Work out the finished part from the listing and answer in its coordinate system (mm). A direction names the side the tool comes from. Coordinates: 2 decimals unless noted, no trailing zeros. Loops run counter-clockwise (first coordinate to the right, second up) from the corner with the lowest first, then second, coordinate; pieces in that order, holes last. Notation, with made-up numbers: (68.5, 87) - (121.5, 87) arc R25 cw to (121.5, 110) - close; hole circle Ø11 at (6, 18.5). An arc over 180 degrees is marked (long way). Write each question's results on one line, items separated by ' | '. Start each with the question number.
Item 1: Section A-A, the plane y = 44 is taken. Write down the section's boundary in (x, z).
Item 2: Consider probe 1 along X at (y, z) = (36, 2.5); probe 2 along Z at (x, y) = (34.5, 22); probe 3 along Y at (x, z) = (28.5, 3.75). Determine where each line is inside the solid, lowest interval first. Write a range as [from, to].
Item 3: Each of these flat-tipped pins is pushed along its axis until it touches: pin 1 Ø6 at (x, y) = (-7, 9) entering from +Z; pin 2 Ø0.9 at (y, z) = (1.5, 3.5) entering from +X; pin 3 Ø0.9 at (y, z) = (1.5, 3.5) entering from -X. Where does it stop, or does it pass through?
Item 4: Section B-B, the plane z = 6 is taken. Write down the section's boundary in (x, y).
Item 5: For a pull along Z with two mould halves and no side action, classify faces 5 (the face through (17, 29, 2)), 6 (the face through (17, 30, 0)), 7 (the face through (17, 58, 3)), 8 (the face through (46, 24, 6)) as +Z half, -Z half, draft (parallel to the pull), parting line (faces both ways), or undercut.
Item 6: Section D-D, the plane z = 1.25 is taken. Write down the section's boundary in (x, y).
Item 7: Section C-C, the plane x = 27 is taken. Write down the section's boundary in (y, z).
Item 8: A tool of negligible diameter and unlimited length cuts with its end or side. For faces 1 (the face through (45, 39, 4.7)), 2 (the face through (0, 2, 3)), 3 (the face through (17, 60, 2)), 4 (the face through (46, 55, 6)), from which of +Z, -Z, +X, -X, +Y, -Y can it reach the whole face along a straight path? Write none if from no direction.
from build123d import *

# Parameters (mm, degrees)
P_IDAT_VYSUNUT_M1_DEPTH = 2
P_IDAT_VYSUNUT_M2_DEPTH = 3
P_IDAT_VYSUNUT_M3_DEPTH = 2


with BuildPart() as part:
    # Skica1 → Přidat vysunutím1 (new body)
    with BuildSketch(Plane.XY):
        Polygon((0, 0), (34, 0), (47, 20), (47, 60), (-13, 60), (-13, 20), align=None)
    extrude(amount=P_IDAT_VYSUNUT_M1_DEPTH)

    # Skica2 → Přidat vysunutím2 (add)
    with BuildSketch(Plane.XY.offset(2)):
        Polygon((-11, 20.592880136), (0, 3.669803213), (0, 0), (-13, 20), (-13, 60), (47, 60), (47, 20), (34, 0), (34, 3.669803213), (45, 20.592880136), (45, 58), (-11, 58), align=None)
    extrude(amount=P_IDAT_VYSUNUT_M2_DEPTH)

    # Skica3 → Přidat vysunutím3 (add)
    with BuildSketch(Plane(origin=(47, 0, 0), x_dir=(0, 0, -1), z_dir=(1, 0, 0))):
        with BuildLine():
            ThreePointArc((-5, 25), (-6, 24), (-7, 25))
            Line((-7, 25), (-7, 54))
            ThreePointArc((-7, 54), (-6, 55), (-5, 54))
            Line((-5, 54), (-5, 56.828427125))
            ThreePointArc((-5, 56.828427125), (-7.732050808, 56.449489743), (-9, 54))
            Line((-9, 54), (-9, 25))
            ThreePointArc((-9, 25), (-7.732050808, 22.550510257), (-5, 22.171572875))
            Line((-5, 22.171572875), (-5, 25))
        make_face()
    extrude(amount=-P_IDAT_VYSUNUT_M3_DEPTH)


solid = part.part
Answer key:
1) outline: (-13, 0) - (47, 0) - (47, 5) - (45, 5) - (45, 2) - (-11, 2) - (-11, 5) - (-13, 5) - close; (45, 7) - (47, 7) - (47, 9) - (45, 9) - close
2) probe 1: x = [-13, -11], [45, 47] | probe 2: z = [0, 2] | probe 3: y = [58, 60]
3) pin 1: stops at z = 5 | pin 2: stops at x = 35.27 | pin 3: stops at x = -1.27
4) outline: (45, 22) - (47, 22) - (47, 24) - (45, 24) - close; (45, 55) - (47, 55) - (47, 57) - (45, 57) - close
5) face 5: +Z half | face 6: -Z half | face 7: draft | face 8: undercut
6) outline: (-13, 20) - (0, 0) - (34, 0) - (47, 20) - (47, 60) - (-13, 60) - close
7) outline: (0, 0) - (60, 0) - (60, 5) - (58, 5) - (58, 2) - (0, 2) - close
8) face 1: +Z | face 2: +Z, -Y | face 3: +Z, -Z, +X, -X, +Y | face 4: +X, -X
